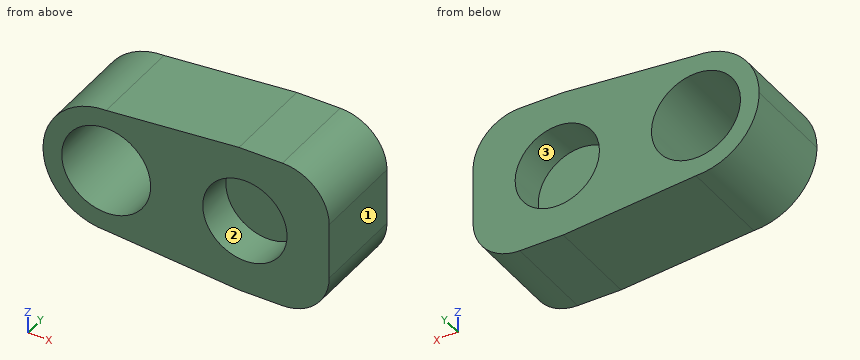
```python
from build123d import *

# Parameters (mm, degrees)
SKETCH1_R           = 4.75
BOSS_EXTRUDE1_DEPTH = 10
SKETCH2_R           = 4.5
CUT_EXTRUDE1_DEPTH  = 4
CUT_EXTRUDE2_START  = -4
SKETCH4_R           = 4.5
CUT_EXTRUDE2_DEPTH  = 4


with BuildPart() as part:
    # Sketch1 → Boss-Extrude1 (new body)
    with BuildSketch(Plane(origin=(0, 0, 0), x_dir=(1, 0, 0), z_dir=(0, 1, 0))):
        with BuildLine():
            Line((5.649139951, 8), (10.28, 8))
            ThreePointArc((10.28, 8), (13.815533906, 6.535533906), (15.28, 3))
            Line((15.28, 3), (15.28, -3))
            ThreePointArc((15.28, -3), (13.815533906, -6.535533906), (10.28, -8))
            Line((10.28, -8), (5.649139951, -8))
            Line((5.649139951, -8), (-8.529960299, -6.75))
            ThreePointArc((-8.529960299, -6.75), (-13.302950922, -4.772978995), (-15.28, 0))
            ThreePointArc((-15.28, 0), (-13.302950922, 4.772978995), (-8.529960299, 6.75))
            Line((-8.529960299, 6.75), (5.649139951, 8))
        make_face()
        with Locations(Location((-8.529960299, 0, 0), (0, 0, 270))):
            Circle(SKETCH1_R, mode=Mode.SUBTRACT)
    extrude(amount=BOSS_EXTRUDE1_DEPTH)

    # Sketch2 → Cut-Extrude1 (cut)
    with BuildSketch(Plane(origin=(0, 10, 0), x_dir=(1, 0, 0), z_dir=(0, 1, 0))):
        with Locations(Location((6.280039701, 0, 0), (0, 0, 270))):
            Circle(SKETCH2_R)
    extrude(amount=-CUT_EXTRUDE1_DEPTH, mode=Mode.SUBTRACT)

    # Sketch4 → Cut-Extrude2 (cut)
    with BuildSketch(Plane.XZ.offset(CUT_EXTRUDE2_START)):
        with Locations(Location((6.280039701, 0, 0), (0, 0, 90))):
            Circle(SKETCH4_R)
    extrude(amount=CUT_EXTRUDE2_DEPTH, mode=Mode.SUBTRACT)


solid = part.part
```
CAD build for the part. Positions are in the model's coordinates, mm. Face numbers are marked on the shaded views. A direction names the side the tool comes from. Round coordinates to 2 decimals unless told otherwise and drop trailing zeros. Order: outer loops, then holes, each group sorted by start corner. A loop starts at its lowest first (then second) coordinate and runs counter-clockwise, first axis right, second up.
Q1. Which spindle directions (+Z, -Z, +X, -X, +Y, -Y) get a long thin tool onto all of the face, cutting with end or side? Do the marked faces 1, 2 and 3. Say none if no direction does.
Q2. Wall check: L1, parallel to X at y = 1.3, z = 0; L2, parallel to X at y = 1.75, z = 2.75; L3, parallel to Y at x = 5.5, z = -3.5. Give the ranges that are in metal, low to high.
Q3. Drop flat-ended pins along their axis: pin 1 (8 mm diameter, centred on x = 5.5, z = -4, fed in from -Y); pin 2 (1.5 mm diameter, centred on x = -10.5, y = 3, fed in from +Z); pin 3 (2.5 mm diameter, centred on x = 7.5, z = -1.5, fed in from +Y); pin 4 (8.5 mm diameter, centred on x = -8.53, z = 0, fed in from -Y). Give the stop position or say it passes through.
Q4. Slice it at A-A (y = 4.5). Write the cut outline in (x, z).
Q5. Slice it at C-C (z = 3.5). Write the cut outline in (x, y).
Q6. Slice it at B-B (x = -9.5). Write the cut outline in (y, z), and give its area (3 significant figures).
Q7. Slice it at D-D (y = 2). Write the cut outline in (x, z).
Results below:
1. face 1: +Z, -Z, +X, +Y, -Y
1. face 2: -Y
1. face 3: +Y
2. L1: x = -15.28 to -13.28, -3.78 to 1.78, 10.78 to 15.28
2. L2: x = -14.69 to -12.4, -4.66 to 2.72, 9.84 to 15.28
2. L3: y = 4 to 6
3. pin 1: stops at y = 0
3. pin 2: stops at z = 6.64
3. pin 3: stops at y = 6
3. pin 4: passes through
4. outline: (-15.28, 0) arc R6.75 ccw to (-8.53, -6.75) - (5.65, -8) - (10.28, -8) arc R5 ccw to (15.28, -3) - (15.28, 3) arc R5 ccw to (10.28, 8) - (5.65, 8) - (-8.53, 6.75) arc R6.75 ccw to start; hole circle Ø9.5 at (-8.53, 0)
5. outline: (-14.3, 0) - (-11.74, 0) - (-11.74, 10) - (-14.3, 10) - close; (-5.32, 0) - (3.45, 0) - (3.45, 4) - (9.11, 4) - (9.11, 0) - (15.25, 0) - (15.25, 10) - (9.11, 10) - (9.11, 6) - (3.45, 6) - (3.45, 10) - (-5.32, 10) - close
6. outline: (0, -6.68) - (10, -6.68) - (10, -4.65) - (0, -4.65) - close; (0, 4.65) - (10, 4.65) - (10, 6.68) - (0, 6.68) - close
6. area: 40.6 mm2
7. outline: (-15.28, 0) arc R6.75 ccw to (-8.53, -6.75) - (5.65, -8) - (10.28, -8) arc R5 ccw to (15.28, -3) - (15.28, 3) arc R5 ccw to (10.28, 8) - (5.65, 8) - (-8.53, 6.75) arc R6.75 ccw to start; hole circle Ø9.5 at (-8.53, 0); hole circle Ø9 at (6.28, 0)
